Solid Edge part; units mm, degrees
sketch "Sketch1" plane through (0, 0, 0) normal (0, -1, 0) x (1, 0, 0)
  line L0 (0, 0) -> (0, 655)
sketch "Sketch2" plane through (0, 0, 0) normal (0, 0, -1) x (-1, 0, 0)
  circle A0 centre (0, 0) radius 12.5
sweep "SweptProtrusion_8" add profiles "Sketch2" path "Sketch1"
sketch "Sketch3" plane through (0, 0, 0) normal (0, -1, 0) x (1, 0, 0)
  arc A0 (0, 655) -> (164, 655) centre (82, 655) cw
sketch "Sketch4" plane through (0, 0, 655) normal (0, 0, 1) x (-1, 0, 0)
  circle A0 centre (0, 0) radius 12.5
sweep "SweptProtrusion_10" add profiles "Sketch4" path "Sketch3"
sketch "Sketch5" plane through (0, 0, 0) normal (0, -1, 0) x (1, 0, 0)
  line L0 (164, 655) -> (164, 0)
sketch "Sketch6" plane through (100, 0, 655) normal (0, 0, -1) x (0, 1, 0)
  circle A0 centre (0, 64) radius 12.5
sweep "SweptProtrusion_11" add profiles "Sketch6" path "Sketch5"
shell "Thinwall_2" thickness 2 removed faces 4 at (8.5833, -8.0833, 0) at (172.5833, -8.0833, 0) at (8.5833, -8.0833, 0) at (172.5833, -8.0833, 0)
properties material "Stainless steel"
Model file for the job. Use its own axes, mm. Round coordinates to 2 decimals unless told otherwise and drop trailing zeros. Order: outer loops, then holes, each group sorted by start corner. A loop starts at its lowest first (then second) coordinate and runs counter-clockwise, first axis right, second up.
(1) Band-saw the part on B-B (z = 221). List the corners of the cut face in (x, y).
(2) Band-saw the part on A-A (y = 0). List the corners of the cut face in (x, z).
(3) Pin check, flat tips, straight feed: pin 1 (1 mm diameter, centred on x = 123.5, y = -2.5, fed in from +Z); pin 2 (5 mm diameter, centred on x = 64.5, y = 6, fed in from -Z) (3 decimals); pin 3 (10 mm diameter, centred on y = 3.5, z = 613.5, fed in from -X); pin 4 (2 mm diameter, centred on y = -7, z = 466.5, fed in from -X). Stop position of each tip, or through.
(4) Drill centre lines: line 1 (X direction, y = 0, z = 63.5); line 2 (X direction, y = -8.75, z = 592); line 3 (Y direction, x = 0, z = 454.5). Where is each one in solid material? Low to high.
Verdict:
1. outline: circle Ø25 at (0, 0); circle Ø25 at (164, 0); hole circle Ø21 at (0, 0); hole circle Ø21 at (164, 0)
2. outline: (-12.5, 0) - (-10.5, 0) - (-10.5, 655) arc R92.5 cw to (174.5, 655) - (174.5, 0) - (176.5, 0) - (176.5, 655) arc R94.5 ccw to (-12.5, 655) - close; (10.5, 0) - (12.5, 0) - (12.5, 655) arc R69.5 cw to (151.5, 655) - (151.5, 0) - (153.5, 0) - (153.5, 655) arc R71.5 ccw to (10.5, 655) - close
3. pin 1: stops at z = 739.89
3. pin 2: stops at z = 722.535
3. pin 3: stops at x = -12.5
3. pin 4: stops at x = -10.97
4. line 1: x = -12.5 to -10.5, 10.5 to 12.5, 151.5 to 153.5, 174.5 to 176.5
4. line 2: x = -8.93 to -5.8, 5.8 to 8.93, 155.07 to 158.2, 169.8 to 172.93
4. line 3: y = -12.5 to -10.5, 10.5 to 12.5
